Geometry: final body of the model. Coordinates: model frame, mm. A direction names the side the tool comes from. Coordinates: 2 decimals unless noted, no trailing zeros. Loops run counter-clockwise (first coordinate to the right, second up) from the corner with the lowest first, then second, coordinate; pieces in that order, holes last. Notation, with made-up numbers: (69, 80) -> (86, 80) arc R13 cw to (86, 86) -> close; hole circle Ø4 at (-24.75, 8). An arc over 180 degrees is marked (long way). One line per item, written item: value. Start each with the question number.
from build123d import *

# Parameters (mm, degrees)
SKETCH_1_R                   = 12.5
EXTRUDE_1_DEPTH              = 15
HOLE_WIZARD_1_D              = 9
HOLE_WIZARD_1_DEPTH          = 100
SKETCH_4_W                   = 53.346686235
SKETCH_4_H                   = 2
CUT_EXTRUDE_1_DEPTH          = 113.722003176
HOLE_WIZARD_M8_1_D           = 8.5
HOLE_WIZARD_M8_1_DEPTH       = 35
HOLE_WIZARD_M8_1_CBORE_D     = 14
HOLE_WIZARD_M8_1_CBORE_DEPTH = 5.5
HOLE_WIZARD_M8_1_TIP         = 2.553657631
CUT_EXTRUDE_2_REACH          = 106.697
SKETCH_8_R                   = 4.5


with BuildPart() as part:
    # 草图1 → 凸台-拉伸1 (new, symmetric)
    with BuildSketch(Plane.XY):
        Polygon((42.5, 0), (-42.5, 0), (-42.5, 12), (-26.5, 12), (-26.5, 100), (26.5, 100), (26.5, 12), (42.5, 12), align=None)
        with Locations((0, 80)):
            Circle(SKETCH_1_R, mode=Mode.SUBTRACT)
    extrude(amount=EXTRUDE_1_DEPTH, both=True)

    # 孔1
    with Locations(Plane.XZ):
        with Locations((-35, 0), (35, 0)):
            Hole(HOLE_WIZARD_1_D / 2, depth=HOLE_WIZARD_1_DEPTH)

    # 草图4 → 切除-拉伸1 (cut, through all)
    with BuildSketch(Plane.XY.offset(15)):
        with Locations((33.672264203, 80)):
            Rectangle(SKETCH_4_W, SKETCH_4_H)
    extrude(amount=-CUT_EXTRUDE_1_DEPTH, mode=Mode.SUBTRACT)

    # M8 六角头螺钉的柱形沉头孔1
    with Locations(Plane(origin=(-72.699544071, 100, 2.28188546), x_dir=(0, 0, -1), z_dir=(0, 1, 0))):
        with Locations((2.28188546, -90.699544071)):
            CounterBoreHole(HOLE_WIZARD_M8_1_D / 2, HOLE_WIZARD_M8_1_CBORE_D / 2, HOLE_WIZARD_M8_1_CBORE_DEPTH, depth=HOLE_WIZARD_M8_1_DEPTH)
            with Locations((0, 0, -(HOLE_WIZARD_M8_1_DEPTH + HOLE_WIZARD_M8_1_TIP / 2))):  # 118° drill point
                Cone(0, HOLE_WIZARD_M8_1_D / 2, HOLE_WIZARD_M8_1_TIP, mode=Mode.SUBTRACT)

    # 草图8 → 切除-拉伸2 (cut, up to next)
    with BuildSketch(Plane(origin=(0, 94.5, 0), x_dir=(1, 0, 0), z_dir=(0, 1, 0)), mode=Mode.PRIVATE) as cut_extrude_2_sk1:
        with Locations(Location((18, 0, 0), (0, 0, 270))):
            Circle(SKETCH_8_R)
    cut_extrude_2_tool1 = extrude(cut_extrude_2_sk1.sketch, amount=-CUT_EXTRUDE_2_REACH, mode=Mode.PRIVATE) & part.part
    add(cut_extrude_2_tool1.solids().sort_by_distance((18, 94.5, 0))[0], mode=Mode.SUBTRACT)


solid = part.part
1. Pin query (flat end, axial travel): pin 1 Ø9 at (y, z) = (56, -0.5) entering from -X; pin 2 Ø5.5 at (y, z) = (89.5, 2) entering from +X; pin 3 Ø4 at (x, z) = (21, 1.5) entering from +Y. Return the tip coordinate at first contact, or that it passes through.
2. Section C-C on x = 8. Return the cut outline in (y, z).
3. Set-up query: faces 1 (the face through (23, 94.5, 0)), 2 (the face through (-26.5, 55, 0)), 3 (the face through (26.5, 46, 0)). Return all of +Z, -Z, +X, -X, +Y, -Y with unobstructed straight access to the full face (end or side cutting, diameter ignored); none if empty.
4. Section D-D on y = 36. Return the cut outline in (x, z).
5. Draft query along Y for faces 4 (the face through (23, 79, 0)), 5 (the face through (-31, 12, 4)), 6 (the face through (23, 81, 0)), 7 (the face through (24.834, 97.288, 1.517)). Return one class per face: released by +Y, released by -Y, zero draft, split by the parting line, or undercut.
6. Line query: L1, parallel to Z at x = 18, y = 68; L2, parallel to Y at x = 23, z = 13; L3, parallel to Y at x = 16, z = -6. Output: solid intervals per line, ascending. Write a range as [from, to].
7. Section B-B on z = 12.75. Return the cut outline in (x, y), plus the area to 3 significant figures.
8. Section A-A on x = 35. Return the cut outline in (y, z), plus the area to 3 significant figures.
Checks:
1. pin 1: x = -26.5
1. pin 2: x = 26.5
1. pin 3: y = 94.5
2. outline: (0, -15) -> (70.4, -15) -> (70.4, 15) -> (0, 15) -> close; (89.6, -15) -> (100, -15) -> (100, 15) -> (89.6, 15) -> close
3. face 1: +Y
3. face 2: +Z, -Z, -X, +Y
3. face 3: +Z, -Z, +X, +Y
4. outline: (-26.5, -15) -> (26.5, -15) -> (26.5, 15) -> (-26.5, 15) -> close
5. face 4: undercut
5. face 5: released by +Y
5. face 6: undercut
5. face 7: zero draft
6. L1: [-15, -4.25], [4.25, 15]
6. L2: [0, 79], [81, 100]
6. L3: [0, 79], [81, 94.5]
7. outline: (-42.5, 0) -> (42.5, 0) -> (42.5, 12) -> (26.5, 12) -> (26.5, 79) -> (12.46, 79) arc R12.5 cw (long way) to (12.46, 81) -> (26.5, 81) -> (26.5, 100) -> (-26.5, 100) -> (-26.5, 12) -> (-42.5, 12) -> close
7. area: 5,170 mm²
8. outline: (0, -15) -> (12, -15) -> (12, -4.5) -> (0, -4.5) -> close; (0, 4.5) -> (12, 4.5) -> (12, 15) -> (0, 15) -> close
8. area: 252 mm²
